```python
from build123d import *

# Parameters (mm, degrees)
BOSS_EXTRUDE1_DEPTH             = 100
CUT_EXTRUDE1_DEPTH              = 115.950260983
CUT_EXTRUDE1_DEPTH_BACK         = 115.950260983
F_6_0MM_DOWEL_HOLE1_D           = 6
F_6_0MM_DOWEL_HOLE1_DEPTH       = 8.197418143
F_6_0MM_DOWEL_HOLE1_CSINK_D     = 6.05
F_6_0MM_DOWEL_HOLE1_CSINK_ANGLE = 90
F_6_0MM_DOWEL_HOLE1_TIP         = 1.802581857
CHAMFER1_SIZE                   = 1.5


with BuildPart() as part:
    # Sketch1 → Boss-Extrude1 (new body)
    with BuildSketch(Plane(origin=(0, 0, 0), x_dir=(0, 0, -1), z_dir=(1, 0, 0))):
        with BuildLine():
            Line((-6, -9.25), (-6, -15.75))
            ThreePointArc((-6, -15.75), (-5.560660172, -16.810660172), (-4.5, -17.25))
            Line((-4.5, -17.25), (23.7, -17.25))
            ThreePointArc((23.7, -17.25), (24.760660172, -16.810660172), (25.2, -15.75))
            Line((25.2, -15.75), (25.2, -8.75))
            ThreePointArc((25.2, -8.75), (25.639339828, -7.689339828), (26.7, -7.25))
            Line((26.7, -7.25), (52.5, -7.25))
            ThreePointArc((52.5, -7.25), (53.560660172, -6.810660172), (54, -5.75))
            Line((54, -5.75), (54, 5.75))
            Line((54, 5.75), (52, 7.75))
            Line((52, 7.75), (23.575260778, 7.75))
            Line((23.575260778, 7.75), (21.787630389, 9.25))
            Line((21.787630389, 9.25), (19.787630389, 9.25))
            Line((19.787630389, 9.25), (18, 7.75))
            Line((18, 7.75), (18, 14.75))
            Line((18, 14.75), (0, 14.75))
            Line((0, 14.75), (0, -10.116025404))
            ThreePointArc((0, -10.116025404), (-0.75, -11.415063509), (-2.25, -11.415063509))
            Line((-2.25, -11.415063509), (-6, -9.25))
        make_face()
    extrude(amount=BOSS_EXTRUDE1_DEPTH)

    # Sketch2 → Cut-Extrude1 (cut, two sides: drawn at the far end of the back side and taken through both)
    with BuildSketch(Plane.XY.offset(-CUT_EXTRUDE1_DEPTH_BACK)):
        Polygon((96.438170518, 14.75), (96.438170518, 4.083333333), (100, -3.916666667), (100, 14.75), align=None)
        Polygon((0, 14.75), (3.561829482, 14.75), (3.561829482, 4.083333333), (0, -3.916666667), align=None)
    extrude(amount=CUT_EXTRUDE1_DEPTH + CUT_EXTRUDE1_DEPTH_BACK, mode=Mode.SUBTRACT)

    # Ø6.0mm Dowel Hole1
    with Locations(Plane(origin=(0, 14.75, 0), x_dir=(1, 0, 0), z_dir=(0, 1, 0))):
        with Locations((15.561829482, 9), (50, 9), (84.438170518, 9)):
            CounterSinkHole(F_6_0MM_DOWEL_HOLE1_D / 2, F_6_0MM_DOWEL_HOLE1_CSINK_D / 2, depth=F_6_0MM_DOWEL_HOLE1_DEPTH, counter_sink_angle=F_6_0MM_DOWEL_HOLE1_CSINK_ANGLE)
            with Locations((0, 0, -(F_6_0MM_DOWEL_HOLE1_DEPTH + F_6_0MM_DOWEL_HOLE1_TIP / 2))):  # 118° drill point
                Cone(0, F_6_0MM_DOWEL_HOLE1_D / 2, F_6_0MM_DOWEL_HOLE1_TIP, mode=Mode.SUBTRACT)

    # Chamfer1
    # the kernel refuses this chamfer: 1.5 mm, written as the material it takes off along each edge
    with BuildSketch(Plane(origin=(84.438170518, 14.75, -9), x_dir=(-1, 0, 0), z_dir=(0, 0, 1))) as chamfer1_piece_1:
        Polygon((3.025 + CHAMFER1_SIZE, 0), (3.025 - CHAMFER1_SIZE * 0.707106781187, CHAMFER1_SIZE * 0.707106781187), (3.025, 0), align=None)
    revolve(axis=Axis((84.438170518, 14.75, -9), (0, -1, 0)), mode=Mode.SUBTRACT)
    with BuildSketch(Plane(origin=(50, 14.75, -9), x_dir=(-1, 0, 0), z_dir=(0, 0, 1))) as chamfer1_piece_2:
        Polygon((3.025 + CHAMFER1_SIZE, 0), (3.025 - CHAMFER1_SIZE * 0.707106781187, CHAMFER1_SIZE * 0.707106781187), (3.025, 0), align=None)
    revolve(axis=Axis((50, 14.75, -9), (0, -1, 0)), mode=Mode.SUBTRACT)
    with BuildSketch(Plane(origin=(15.561829482, 14.75, -9), x_dir=(-1, 0, 0), z_dir=(0, 0, 1))) as chamfer1_piece_3:
        Polygon((3.025 + CHAMFER1_SIZE, 0), (3.025 - CHAMFER1_SIZE * 0.707106781187, CHAMFER1_SIZE * 0.707106781187), (3.025, 0), align=None)
    revolve(axis=Axis((15.561829482, 14.75, -9), (0, -1, 0)), mode=Mode.SUBTRACT)


solid = part.part
```
Source: CAD feature listing. Evaluate the final solid. Frame: model axes, mm. A direction names the side the tool comes from. Coordinates: 2 decimals unless noted, no trailing zeros. Loops run counter-clockwise (first coordinate to the right, second up) from the corner with the lowest first, then second, coordinate; pieces in that order, holes last. Notation, with made-up numbers: M 40.25,-27 L 95.25,-27 A10 cw 95.25,-12 Z; hole C -9.75,89 d3. An arc over 180 degrees is marked long. Put each result on its own line as item: value. Start each with the question number.
1) Reachability of faces 5 (the face through (49.3, -10.348, 4.099)), 6 (the face through (49, -7.25, -39)), 7 (the face through (49, 7.75, -38)), 8 (the face through (84.054, 5.063, -9.352)), 9 (the face through (96.438, 8, -21)) from +Z, -Z, +X, -X, +Y, -Y: full face, straight path, thin tool, end or side. Return the list, or none.
2) Cut plane D-D on y = 2.5. Return the cut outline in (x, z).
3) Cut plane B-B on z = -34. Return the cut outline in (x, y).
4) Cut plane A-A on x = 91. Return the cut outline in (y, z).
5) Cut plane C-C on y = -13.5. Return the cut outline in (x, z).
6) Ray query, L1, parallel to X at y = 8, z = -9; L2, parallel to Z at x = 84.5, y = 9; L3, parallel to X at y = 8.5, z = -8. Return the intervals inside material, ascending. Write a range as from..to.
7) Pull-direction query (Z, two-part tool) for faces 1 (the face through (53, 10, -9)), 2 (the face through (100, -10, -17)), 3 (the face through (49, -12, 6)), 4 (the face through (18.56, 10.28, -9.13)); classes: pulls with the +Z half, pulls with the -Z half, needs draft (parallel to the pull), parting line crosses it, or undercut.
8) Contact query for flat-ended pins moving along their axis: pin 1 Ø8.5 at (x, z) = (54.5, -41.5) entering from +Y; pin 2 Ø1 at (x, y) = (54.5, 11) entering from +Z; pin 3 Ø1 at (x, z) = (59.5, -21) entering from +Y. Output: stop coordinate, or through.
The answers:
1. face 5: +X, -X, +Y
1. face 6: -Z, +X, -X, -Y
1. face 7: -Z, +X, -X, +Y
1. face 8: +Y
1. face 9: +Z, -Z, +X, +Y
2. outline: M 2.86,-54 L 97.14,-54 L 97.14,0 L 2.86,0 Z
3. outline: M 0,-7.25 L 100,-7.25 L 100,-3.92 L 96.44,4.08 L 96.44,7.75 L 3.56,7.75 L 3.56,4.08 L 0,-3.92 Z
4. outline: M -17.25,-23.7 A1.5 ccw -15.75,-25.2 L -8.75,-25.2 A1.5 cw -7.25,-26.7 L -7.25,-52.5 A1.5 ccw -5.75,-54 L 5.75,-54 L 7.75,-52 L 7.75,-23.58 L 9.25,-21.79 L 9.25,-19.79 L 7.75,-18 L 14.75,-18 L 14.75,0 L -10.12,0 A1.5 cw -11.42,2.25 L -9.25,6 L -15.75,6 A1.5 ccw -17.25,4.5 Z
5. outline: M 0,-25.2 L 100,-25.2 L 100,6 L 0,6 Z
6. L1: x = 3.56..12.56, 18.56..47, 53..81.44, 87.44..96.44
6. L2: z = -22.09..-19.49, -18..-12, -6..0
6. L3: x = 3.56..12.73, 18.39..47.17, 52.83..81.61, 87.27..96.44
7. face 1: undercut
7. face 2: needs draft
7. face 3: pulls with the +Z half
7. face 4: undercut
8. pin 1: stops at y = 7.75
8. pin 2: stops at z = 0
8. pin 3: stops at y = 9.25
